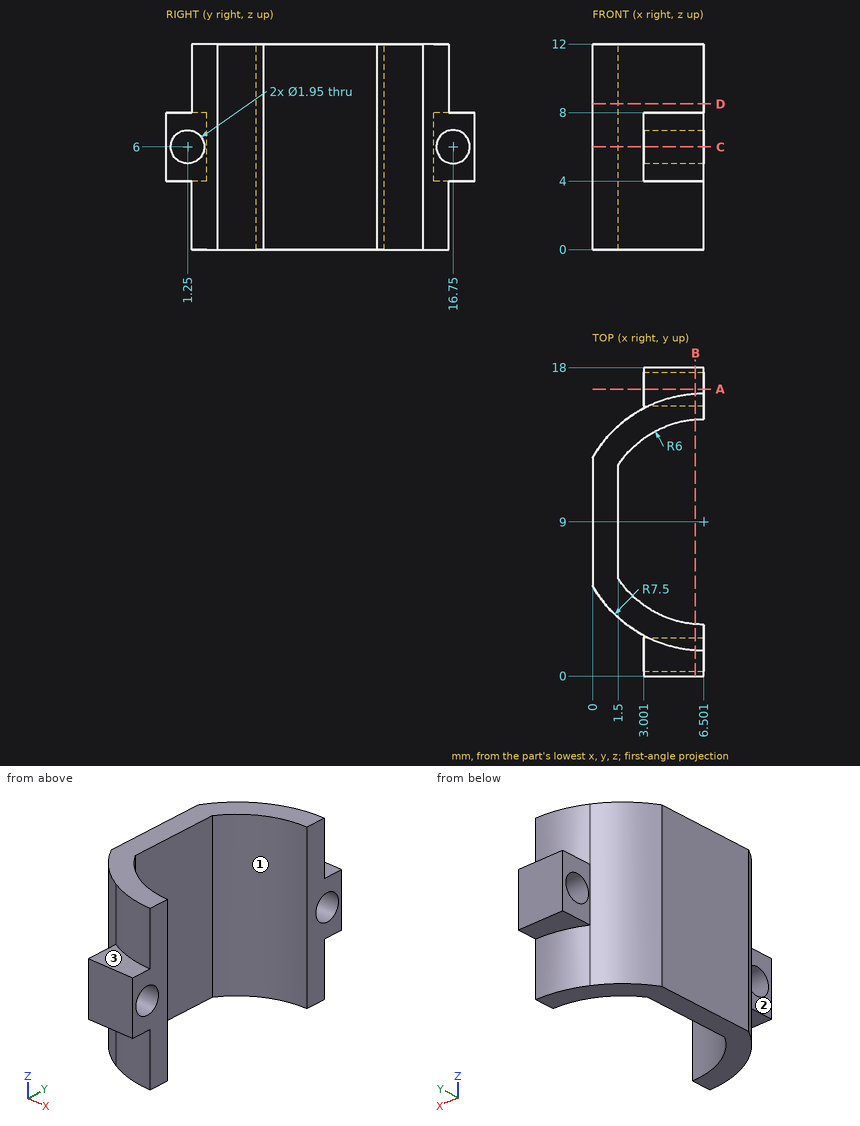
Source: three-view drawing plus pictorial views. Frame: mm from the lowest corner of the part. A direction names the side the tool comes from. Coordinates: 2 decimals unless noted, no trailing zeros. Write each loop counter-clockwise with the first axis right and the second up, starting at its lowest first coordinate (ties: lowest second). Pieces come first, ordered by that corner, then holes. Notation, with made-up numbers: (28.5, 60.5) -> (71.5, 60.5) arc R31 cw to (71.5, 93.5) -> close; hole circle Ø1 at (-24.75, -21). An arc over 180 degrees is marked (long way). Answer as a JSON object with one key per item and string values.
1. Section D-D on z = 8.5. Return the cut outline in (x, y) (3 decimals).
Result set:
{"outline": "(0, 5.26) arc R7.5 ccw to (6.501, 1.5) -> (6.501, 3) arc R6 cw to (1.5, 5.685) -> (1.5, 12.315) arc R6 cw to (6.501, 15) -> (6.501, 16.5) arc R7.5 ccw to (0, 12.74) -> close"}
2. Section B-B on x = 6. Return the cut outline in (y, z) (3 decimals).
Result set:
{"outline": "(0, 4) -> (1.517, 4) -> (1.517, 0) -> (3.021, 0) -> (3.021, 12) -> (1.517, 12) -> (1.517, 8) -> (0, 8) -> close; (14.979, 0) -> (16.483, 0) -> (16.483, 4) -> (18, 4) -> (18, 8) -> (16.483, 8) -> (16.483, 12) -> (14.979, 12) -> close; hole circle Ø1.95 at (1.25, 6); hole circle Ø1.95 at (16.75, 6)"}
3. Section C-C on z = 6. Return the cut outline in (x, y) (3 decimals).
Result set:
{"outline": "(0, 5.26) arc R7.5 ccw to (3.001, 2.367) -> (3.001, 2.225) -> (6.501, 2.225) -> (6.501, 3) arc R6 cw to (1.5, 5.685) -> (1.5, 12.315) arc R6 cw to (6.501, 15) -> (6.501, 15.775) -> (3.001, 15.775) -> (3.001, 15.633) arc R7.5 ccw to (0, 12.74) -> close; (3.001, 0) -> (6.501, 0) -> (6.501, 0.275) -> (3.001, 0.275) -> close; (3.001, 17.725) -> (6.501, 17.725) -> (6.501, 18) -> (3.001, 18) -> close"}
4. Material intervals for line 1 (Y direction, x = 5.65, z = 6) (1 decimal); line 2 (Y direction, x = 3.8, z = 6) (1 decimal); line 3 (X direction, y = 9.75, z = 4.75), sorted ascending. Write a range as from..to.
Result set:
{"line 1": "y = 0..0.3, 2.2..3.1, 14.9..15.8, 17.7..18", "line 2": "y = 0..0.3, 2.2..3.6, 14.4..15.8, 17.7..18", "line 3": "x = 0..1.5"}
5. First-contact query: P1, Ø1.5, axis at x = 2, z = 9, coming from the +Y side; P2, Ø1, axis at x = 6, z = 10, coming from the -Y side; P3, Ø3, axis at y = 1.25, z = 6, coming from the -X side (1 decimal). Flat tips, straight axial feed; report the tip coordinate or a pass-through.
Result set:
{"P1": "stops at y = 15.49", "P2": "stops at y = 1.5", "P3": "stops at x = 2.4"}
6. Access query for the marked faces 1, 2 and 3. Directions: +Z, -Z, +X, -X, +Y, -Y. A direction counts if a zero-diameter tool reaches every point of the face in a straight line with its end or side. Return the directions, or none.
Result set:
{"face 1": "+Z, -Z, +X", "face 2": "+Z, -Z, -X, -Y", "face 3": "+Z, -X, -Y"}
7. Section A-A on y = 16.75. Return the cut outline in (x, z) (3 decimals).
Result set:
{"outline": "(3.001, 4) -> (6.501, 4) -> (6.501, 5.025) -> (3.001, 5.025) -> close; (3.001, 6.975) -> (6.501, 6.975) -> (6.501, 8) -> (3.001, 8) -> close"}
